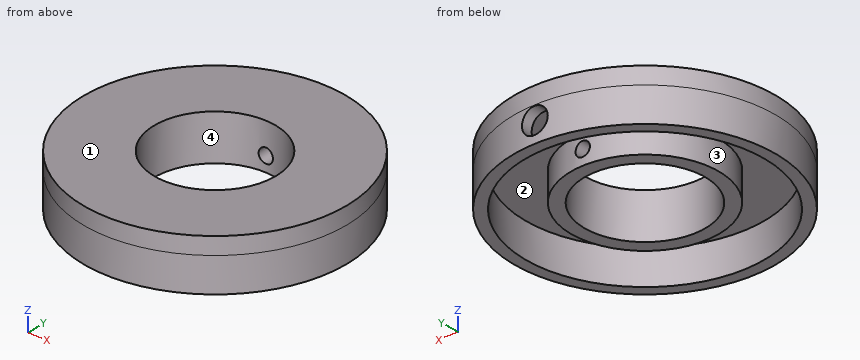
```python
from build123d import *

# Parameters (mm, degrees)
SKETCH1_R           = 23
SKETCH1_R_2         = 10.62
BOSS_EXTRUDE1_DEPTH = 3
BOSS_EXTRUDE3_START = -8
SKETCH2_R           = 13
SKETCH2_R_2         = 10.62
BOSS_EXTRUDE3_DEPTH = 8
BOSS_EXTRUDE4_START = 6
SKETCH3_R           = 23
SKETCH3_R_2         = 21
BOSS_EXTRUDE4_DEPTH = 6
SKETCH4_R           = 1.25
CUT_EXTRUDE1_DEPTH  = 17
SKETCH4_3_R         = 2.25
CUT_EXTRUDE2_DEPTH  = 7


with BuildPart() as part:
    # Sketch1 → Boss-Extrude1 (new body)
    with BuildSketch(Plane.XY):
        Circle(SKETCH1_R)
        Circle(SKETCH1_R_2, mode=Mode.SUBTRACT)
    extrude(amount=BOSS_EXTRUDE1_DEPTH)

    # Sketch2 → Boss-Extrude3 (add)
    with BuildSketch(Plane.XY.offset(3).offset(BOSS_EXTRUDE3_START)):
        Circle(SKETCH2_R)
        Circle(SKETCH2_R_2, mode=Mode.SUBTRACT)
    extrude(amount=BOSS_EXTRUDE3_DEPTH)

    # Sketch3 → Boss-Extrude4 (add)
    with BuildSketch(Plane(origin=(0, 0, 0), x_dir=(-1, 0, 0), z_dir=(0, 0, -1)).offset(BOSS_EXTRUDE4_START)):
        Circle(SKETCH3_R)
        Circle(SKETCH3_R_2, mode=Mode.SUBTRACT)
    extrude(amount=-BOSS_EXTRUDE4_DEPTH)

    # Sketch4 → Cut-Extrude1 (cut)
    with BuildSketch(Plane(origin=(0, 24.918884167, 0), x_dir=(1, 0, 0), z_dir=(0, 1, 0))):
        with Locations(Location((0, 2.407178774, 0), (0, 0, 270))):
            Circle(SKETCH4_R)
    extrude(amount=-CUT_EXTRUDE1_DEPTH, mode=Mode.SUBTRACT)

    # Sketch4_3 → Cut-Extrude2 (cut)
    with BuildSketch(Plane(origin=(0, 24.918884167, 0), x_dir=(1, 0, 0), z_dir=(0, 1, 0))):
        with Locations(Location((0, 2.407178774, 0), (0, 0, 270))):
            Circle(SKETCH4_3_R)
    extrude(amount=-CUT_EXTRUDE2_DEPTH, mode=Mode.SUBTRACT)


solid = part.part
```
The model under review builds one solid part; all positions refer to its coordinate system, in mm. Face numbers are marked on the shaded views. A direction names the side the tool comes from. Give positions to 0.01 mm unless a question says otherwise; leave off trailing zeros. Loops run counter-clockwise (first coordinate to the right, second up) from the corner with the lowest first, then second, coordinate; pieces in that order, holes last. Notation, with made-up numbers: (1.5, 80) -> (7.5, 80) arc R18 cw to (7.5, 106) -> close; hole circle Ø4 at (76, -8.5). An arc over 180 degrees is marked (long way). Use CSV: the item, a comma, the result in double quotes.
1. Consider section B-B, the plane x = 0. Write out the cut boundary in (y, z).
Result:
outline,"(-23, -6) -> (-21, -6) -> (-21, 0) -> (-13, 0) -> (-13, -5) -> (-10.62, -5) -> (-10.62, 3) -> (-23, 3) -> close; (10.62, -5) -> (13, -5) -> (13, -3.66) -> (10.62, -3.66) -> close; (10.62, -1.16) -> (13, -1.16) -> (13, 0) -> (21, 0) -> (21, -0.16) -> (23, -0.16) -> (23, 3) -> (10.62, 3) -> close; (21, -6) -> (23, -6) -> (23, -4.66) -> (21, -4.66) -> close"
2. Machinability: for the marked faces 3 and 4, which of the approach directions +Z, -Z, +X, -X, +Y, -Y give a long, thin tool a straight path to every point of the face, cutting with its end or side? Answer none if there is none.
Result:
face 3,"-Z"
face 4,"+Z, -Z"
3. Consider section C-C, the plane z = -2.5. Write out the cut boundary in (x, y), then the cut area to 3 significant figures.
Result:
outline,"(-2.25, 20.88) -> (-2.25, 22.89) arc R23 ccw (long way) to (2.25, 22.89) -> (2.25, 20.88) arc R21 cw (long way) to start; (-1.25, 10.55) -> (-1.25, 12.94) arc R13 ccw (long way) to (1.25, 12.94) -> (1.25, 10.55) arc R10.62 cw (long way) to start"
area,"438 mm²"
4. To check wall thickness, follow probe 1 along Z at (x, y) = (0, 12); probe 2 along Y at (x, z) = (0, -1.5); probe 3 along Y at (x, z) = (9.5, -1.75). State the ranges of each line that lie inside material, in increasing order. Write a range as from..to.
Result:
probe 1,"z = -5..-3.66, -1.16..3"
probe 2,"y = -23..-21, -13..-10.62"
probe 3,"y = -20.95..-18.73, -8.87..-4.75, 4.75..8.87, 18.73..20.95"
5. The part is to be moulded in two halves that separate along X. For the marked faces 1 and 2, say which applies: +X half, -X half, draft (parallel to the pull), parting line (faces both ways), or undercut.
Result:
face 1,"draft"
face 2,"undercut"
6. For P1, Ø4, axis at y = 4.5, z = 1.5, coming from the -X side; P2, Ø3, axis at x = -13.5, z = 0.5, coming from the -Y side; P3, Ø21, axis at x = 1.5, y = 1, coming from the -Z side; P4, Ø12, axis at x = 10, y = 3.5, coming from the +Z side, all flat-tipped, find the tip position at first contact; note any pin that passes through.
Result:
P1,"stops at x = -22.86"
P2,"stops at y = -19.62"
P3,"stops at z = -5"
P4,"stops at z = 3"
7. Consider section D-D, the plane x = -10. Write out the cut boundary in (y, z), then the cut area to 3 significant figures.
Result:
outline,"(-20.71, -6) -> (-18.47, -6) -> (-18.47, 0) -> (-8.31, 0) -> (-8.31, -5) -> (-3.58, -5) -> (-3.58, 3) -> (-20.71, 3) -> close; (3.58, -5) -> (8.31, -5) -> (8.31, 0) -> (18.47, 0) -> (18.47, -6) -> (20.71, -6) -> (20.71, 3) -> (3.58, 3) -> close"
area,"177 mm²"
8. Consider section A-A, the plane y = 0. Write out the cut boundary in (x, z).
Result:
outline,"(-23, -6) -> (-21, -6) -> (-21, 0) -> (-13, 0) -> (-13, -5) -> (-10.62, -5) -> (-10.62, 3) -> (-23, 3) -> close; (10.62, -5) -> (13, -5) -> (13, 0) -> (21, 0) -> (21, -6) -> (23, -6) -> (23, 3) -> (10.62, 3) -> close"
